Geometry check sheet. Reference: the model listing, model coordinates, mm. Face numbers are marked on the shaded views. A direction names the side the tool comes from. Coordinates: 2 decimals unless noted, no trailing zeros. Write each loop counter-clockwise with the first axis right and the second up, starting at its lowest first coordinate (ties: lowest second). Pieces come first, ordered by that corner, then holes. Notation, with made-up numbers: (17, 30.25) -> (64, 30.25) arc R20 ccw to (64, 43.25) -> close; hole circle Ø2 at (8, 81). An arc over 180 degrees is marked (long way). Use a Markdown table: item, result.
Solid Edge part; units mm, degrees
sketch "Sketch1" plane through (0, 0, 0) normal (1, 0, 0) x (0, 1, 0)
  line L0 (-38, 10) -> (-45, -10)
  line L1 (-45, -10) -> (45, -10)
  line L2 (38, 10) -> (45, -10)
  line L3 (38, 10) -> (-38, 10)
extrude "Protrusion1" add sketch "Sketch1" along normal mid plane 60
sketch "Sketch2" plane through (0, 0, 0) normal (1, 0, 0) x (0, 1, 0)
  line L0 (-25, 48) -> (-38, 10)
  line L1 (-38, 10) -> (38, 10)
  line L2 (25, 48) -> (38, 10)
  line L3 (25, 48) -> (-25, 48)
extrude "ExtrudedProtrusion_2" add sketch "Sketch2" along normal mid plane 24
sketch "Sketch3" plane through (0, 0, 0) normal (1, 0, 0) x (0, 1, 0)
  circle A0 centre (0, 40) radius 20
extrude "ExtrudedProtrusion_3" add sketch "Sketch3" along normal mid plane 44
sketch "Sketch4" plane through (0, 0, 0) normal (1, 0, 0) x (0, 1, 0)
  line L0 (-41.85, 35) -> (-41.85, -1)
  line L1 (-41.85, -1) -> (41.85, -1)
  line L2 (41.85, -1) -> (41.85, 35)
  line L3 (41.85, 35) -> (-41.85, 35)
extrude "ExtrudedProtrusion_4" add sketch "Sketch4" along normal mid plane 16
sketch "Sketch5" plane through (0, 0, 0) normal (1, 0, 0) x (0, 1, 0)
  circle A0 centre (0, 40) radius 8
extrude "ExtrudedCutout_1" cut sketch "Sketch5" along normal mid plane 44
sketch "Sketch6" plane through (0, -21.6652, 48) normal (0, 0, 1) x (1, 0, 0)
  line L0 (-12, 13.6652) -> (-12, -3.3348)
  line L1 (-12, -3.3348) -> (12, -3.3348)
  line L2 (12, -3.3348) -> (12, 13.6652)
  line L3 (12, 13.6652) -> (-12, 13.6652)
extrude "ExtrudedCutout_2" cut sketch "Sketch6" along normal blind 20.2451
mirror "Mirror1" about plane through (0, 0, 0) normal (0, -1, 0) of "ExtrudedCutout_2"
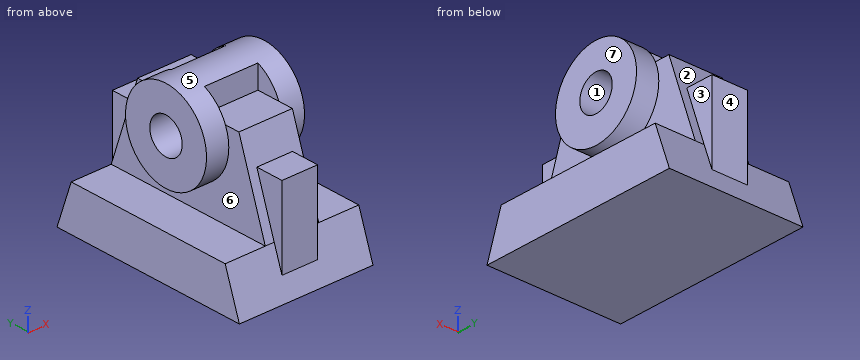
Item 1: Section check D-D on z = 40. Record the boundary of the cut face in (x, y).
Answer block:
| item | result |
|---|---|
| outline | (-22, -20) -> (-12, -20) -> (-12, -27.74) -> (12, -27.74) -> (12, -20) -> (22, -20) -> (22, -8) -> (-22, -8) -> close; (-22, 8) -> (22, 8) -> (22, 20) -> (12, 20) -> (12, 27.74) -> (-12, 27.74) -> (-12, 20) -> (-22, 20) -> close |
Item 2: Mould release check, pull along Z, two halves, no side actions. Record for the marked faces 1, 2 and 3: +Z half, -Z half, draft (parallel to the pull), parting line (faces both ways), or undercut.
Answer block:
| item | result |
|---|---|
| face 1 | undercut |
| face 2 | +Z half |
| face 3 | draft |
Item 3: Section check C-C on x = 0. Record the boundary of the cut face in (y, z).
Answer block:
| item | result |
|---|---|
| outline | (-45, -10) -> (45, -10) -> (41.85, -1) -> (41.85, 35) -> (29.45, 35) -> (25, 48) -> (8, 48) -> (8, 58.33) arc R20 ccw to (-8, 58.33) -> (-8, 48) -> (-25, 48) -> (-29.45, 35) -> (-41.85, 35) -> (-41.85, -1) -> close; hole circle Ø16 at (0, 40) |
Item 4: Thickness scan on L1, parallel to Z at x = 13.5, y = 0; L2, parallel to Z at x = 9, y = 0; L3, parallel to Y at x = 0, z = 50.5. Record the ranges inside material, lowest first. Write a range as [from, to].
Answer block:
| item | result |
|---|---|
| L1 | z = [-10, 10], [20, 32], [48, 60] |
| L2 | z = [-10, 32], [48, 60] |
| L3 | y = [-8, 8] |
Item 5: Tool access check on the marked faces 4, 5, 6 and 7. Record the directions out of +Z, -Z, +X, -X, +Y, -Y that give a thin tool (end or side, any length) a straight path to the whole face; none if there is none.
Answer block:
| item | result |
|---|---|
| face 4 | +Z, +X, -X, +Y |
| face 5 | none |
| face 6 | -X |
| face 7 | +Z, +X, +Y, -Y |
Item 6: Section check B-B on z = 7. Record the boundary of the cut face in (x, y).
Answer block:
| item | result |
|---|---|
| outline | (-30, -39.05) -> (-8, -39.05) -> (-8, -41.85) -> (8, -41.85) -> (8, -39.05) -> (30, -39.05) -> (30, 39.05) -> (8, 39.05) -> (8, 41.85) -> (-8, 41.85) -> (-8, 39.05) -> (-30, 39.05) -> close |
Item 7: Section check A-A on y = 0. Record the boundary of the cut face in (x, z).
Answer block:
| item | result |
|---|---|
| outline | (-30, -10) -> (30, -10) -> (30, 10) -> (12, 10) -> (12, 20) -> (22, 20) -> (22, 32) -> (-22, 32) -> (-22, 20) -> (-12, 20) -> (-12, 10) -> (-30, 10) -> close; (-22, 48) -> (22, 48) -> (22, 60) -> (-22, 60) -> close |
Item 8: Depth check by flat-ended pin: P1, Ø2, axis at x = -14, z = 14.5, coming from the +Y side; P2, Ø5, axis at x = 3.5, z = 19, coming from the -Y side; P3, Ø5, axis at y = 13, z = 51.5, coming from the -X side; P4, Ø12, axis at x = 11, z = 48.5, coming from the -Y side. Enter the tip coordinate at first touch or a pass-through.
Answer block:
| item | result |
|---|---|
| P1 | passes through |
| P2 | stops at y = -41.85 |
| P3 | stops at x = -22 |
| P4 | stops at y = -26.88 |
